from build123d import *

# Parameters (mm, degrees)
SKETCH1_W           = 126
SKETCH1_H           = 90
BOSS_EXTRUDE1_DEPTH = 3
BOSS_EXTRUDE2_DEPTH = 177
SKETCH3_W           = 126
SKETCH3_H           = 90
BOSS_EXTRUDE3_DEPTH = 3
FILLET1_R           = 10
SKETCH5_R           = 3
CUT_EXTRUDE1_DEPTH  = 5
SKETCH6_W           = 22.5
SKETCH6_H           = 13.5
SKETCH6_W_2         = 15
SKETCH6_H_2         = 10
CUT_EXTRUDE2_DEPTH  = 3
SKETCH7_W           = 180
SKETCH7_H           = 180
BOSS_EXTRUDE5_DEPTH = 3
SKETCH8_OUTSIDE_W   = 236
SKETCH8_OUTSIDE_H   = 146
CUT_EXTRUDE3_DEPTH  = 181
SKETCH9_W           = 120
SKETCH9_H           = 87
CUT_EXTRUDE4_DEPTH  = 181
SKETCH11_W          = 10
SKETCH11_H          = 3
BOSS_EXTRUDE6_DEPTH = 10
SKETCH12_R          = 1.7
CUT_EXTRUDE5_DEPTH  = 10
SKETCH13_R          = 1.7
CUT_EXTRUDE6_DEPTH  = 10
SKETCH16_W          = 60
SKETCH16_H          = 45
SKETCH16_W_2        = 55.136481679
SKETCH16_H_2        = 30
SKETCH16_W_3        = 50
SKETCH16_W_4        = 57.73113964
SKETCH16_W_5        = 14.594951033
SKETCH16_W_6        = 24.912721932
SKETCH16_H_3        = 36.48422414
BOSS_EXTRUDE7_DEPTH = 5
SKETCH15_R          = 4.75
SKETCH15_R_2        = 3
SKETCH15_R_3        = 3.6
SKETCH15_R_4        = 4.6
SKETCH15_R_5        = 4.7
SKETCH15_W          = 22.5
SKETCH15_H          = 13.5
CUT_EXTRUDE7_DEPTH  = 7.5
FILLET3_R           = 2.27
SKETCH17_W          = 54
SKETCH17_H          = 180
CUT_EXTRUDE8_DEPTH  = 10
BOSS_EXTRUDE8_DEPTH = 2
SKETCH19_R          = 1.7
CUT_EXTRUDE9_DEPTH  = 12
SKETCH20_R          = 1.7
CUT_EXTRUDE10_DEPTH = 12


with BuildPart() as part:
    # Sketch1 → Boss-Extrude1 (new body)
    with BuildSketch(Plane.XY):
        with Locations((63, -45)):
            Rectangle(SKETCH1_W, SKETCH1_H)
    extrude(amount=BOSS_EXTRUDE1_DEPTH)

    # Sketch2 → Boss-Extrude2 (add)
    with BuildSketch(Plane(origin=(0, 0, 0), x_dir=(-1, 0, 0), z_dir=(0, 0, -1))):
        Polygon((-126, -90), (-126, 0), (0, 0), (0, -90), (-3, -90), (-3, -3), (-123, -3), (-123, -90), align=None)
    extrude(amount=-BOSS_EXTRUDE2_DEPTH)

    # Sketch3 → Boss-Extrude3 (add)
    with BuildSketch(Plane.XY.offset(177)):
        with Locations((63, -45)):
            Rectangle(SKETCH3_W, SKETCH3_H)
    extrude(amount=BOSS_EXTRUDE3_DEPTH)

    # Fillet1
    fillet1_edges = [part.edges().sort_by_distance(p)[0] for p in [
        (63, -3, 3),
        (63, -3, 177),
        (63, 0, 0),
        (63, 0, 180),
    ]]
    fillet(fillet1_edges, radius=FILLET1_R)

    # Sketch5 → Cut-Extrude1 (cut)
    with BuildSketch(Plane.ZY.offset(2)):
        with Locations((154.879918412, -80.109384213)):
            Circle(SKETCH5_R)
        with Locations((163.20022023, -80.109384213)):
            Circle(SKETCH5_R)
    extrude(amount=-CUT_EXTRUDE1_DEPTH, mode=Mode.SUBTRACT)

    # Sketch6 → Cut-Extrude2 (cut)
    with BuildSketch(Plane(origin=(126, 0, 0), x_dir=(0, 0, -1), z_dir=(1, 0, 0))):
        with Locations((-31.25, -25.595398102)):
            Rectangle(SKETCH6_W, SKETCH6_H)
        with Locations((-30.5, -72.125177246)):
            Rectangle(SKETCH6_W_2, SKETCH6_H_2)
    extrude(amount=-CUT_EXTRUDE2_DEPTH, mode=Mode.SUBTRACT)

    # Sketch7 → Boss-Extrude5 (add)
    with BuildSketch(Plane(origin=(0, -90, 0), x_dir=(-1, 0, 0), z_dir=(0, -1, 0))):
        with Locations((-90, -90)):
            Rectangle(SKETCH7_W, SKETCH7_H)
    extrude(amount=-BOSS_EXTRUDE5_DEPTH)

    # Sketch8 outside → Cut-Extrude3 (cut, through all)
    with BuildSketch(Plane.ZY):
        with Locations((90, -45)):
            Rectangle(SKETCH8_OUTSIDE_W, SKETCH8_OUTSIDE_H)
        with BuildLine():
            Line((0, -79.898662722), (0, -90))
            Line((0, -90), (10.101337278, -90))
            Line((10.101337278, -90), (169.898662722, -90))
            Line((169.898662722, -90), (180, -90))
            Line((180, -90), (180, -79.898662722))
            Line((180, -79.898662722), (180, -10.101337278))
            ThreePointArc((180, -10.101337278), (177.04138681, -2.95861319), (169.898662722, 0))
            Line((169.898662722, 0), (10.101337278, 0))
            ThreePointArc((10.101337278, 0), (2.95861319, -2.95861319), (0, -10.101337278))
            Line((0, -10.101337278), (0, -79.898662722))
        make_face(mode=Mode.SUBTRACT)
    extrude(amount=-CUT_EXTRUDE3_DEPTH, mode=Mode.SUBTRACT)

    # Sketch9 → Cut-Extrude4 (cut, through all)
    with BuildSketch(Plane(origin=(0, 0, 0), x_dir=(-1, 0, 0), z_dir=(0, 0, -1))):
        with Locations((-63, -43.5)):
            Rectangle(SKETCH9_W, SKETCH9_H)
    extrude(amount=-CUT_EXTRUDE4_DEPTH, mode=Mode.SUBTRACT)

    # Sketch11 → Boss-Extrude6 (add)
    with BuildSketch(Plane(origin=(0, -87, 0), x_dir=(1, 0, 0), z_dir=(0, 1, 0))):
        with Locations((38, -178.5)):
            Rectangle(SKETCH11_W, SKETCH11_H)
        with Locations((88, -178.5)):
            Rectangle(SKETCH11_W, SKETCH11_H)
        with Locations((38, -1.5)):
            Rectangle(SKETCH11_W, SKETCH11_H)
        with Locations((88, -1.5)):
            Rectangle(SKETCH11_W, SKETCH11_H)
    extrude(amount=BOSS_EXTRUDE6_DEPTH)

    # Sketch12 → Cut-Extrude5 (cut)
    with BuildSketch(Plane(origin=(0, 0, 0), x_dir=(-1, 0, 0), z_dir=(0, 0, -1))):
        with Locations((-88, -82)):
            Circle(SKETCH12_R)
        with Locations((-38, -82)):
            Circle(SKETCH12_R)
    extrude(amount=-CUT_EXTRUDE5_DEPTH, mode=Mode.SUBTRACT)

    # Sketch13 → Cut-Extrude6 (cut)
    with BuildSketch(Plane.XY.offset(180)):
        with Locations((38, -82)):
            Circle(SKETCH13_R)
        with Locations((88, -82)):
            Circle(SKETCH13_R)
    extrude(amount=-CUT_EXTRUDE6_DEPTH, mode=Mode.SUBTRACT)

    # Sketch16 → Boss-Extrude7 (add)
    with BuildSketch(Plane.ZY.offset(2)):
        with Locations((33.397799687, -29.5)):
            Rectangle(SKETCH16_W, SKETCH16_H)
        with Locations((33.81824084, -70)):
            Rectangle(SKETCH16_W_2, SKETCH16_H_2)
        with Locations((93.535533906, -30.5)):
            Rectangle(SKETCH16_W_3, SKETCH16_H)
        with Locations((92.012227586, -70)):
            Rectangle(SKETCH16_W_4, SKETCH16_H_2)
        with Locations((130.607764761, -69.962221636)):
            Rectangle(SKETCH16_W_5, SKETCH16_H_2)
        with Locations((165.153259598, -44.347490411)):
            Rectangle(SKETCH16_W_6, SKETCH16_H_3)
    extrude(amount=-BOSS_EXTRUDE7_DEPTH)

    # Sketch15 → Cut-Extrude7 (cut, symmetric)
    with BuildSketch(Plane.ZY.offset(2)):
        with Locations((11.897799687, -25)):
            Circle(SKETCH15_R)
        with Locations((35.120412136, -25)):
            Circle(SKETCH15_R_2)
        with Locations((55.547244011, -25)):
            Circle(SKETCH15_R_3)
        with Locations((93.316630751, -36.188493445)):
            Circle(SKETCH15_R_4)
        with Locations((12.826376296, -70.752206375)):
            Circle(SKETCH15_R_3)
        with Locations((54.826376296, -70.752206375)):
            Circle(SKETCH15_R_3)
        with Locations((34.603168291, -70.752206375)):
            Circle(SKETCH15_R_4)
        with Locations((35.201614473, -42.050293137)):
            Circle(SKETCH15_R_4)
        with Locations((112.872652377, -74.126778902)):
            Circle(SKETCH15_R_3)
        with Locations((130.71133323, -74.126778902)):
            Circle(SKETCH15_R_3)
        with Locations((139.753590628, -46.167682179)):
            Circle(SKETCH15_R_5)
        with Locations((165.243179484, -54.550293137)):
            Circle(SKETCH15_R_3)
        with Locations((165.243179484, -38.990832132)):
            Circle(SKETCH15_R_2)
        with Locations((84.43777437, -74.416080578)):
            Rectangle(SKETCH15_W, SKETCH15_H)
    extrude(amount=CUT_EXTRUDE7_DEPTH, both=True, mode=Mode.SUBTRACT)

    # Fillet3
    fillet3_edges = [part.edges().sort_by_distance(p)[0] for p in [
        (-1, -52, 3.397799687),
        (-1, -7, 3.397799687),
        (-1, -7, 63.397799687),
        (-1, -52, 63.397799687),
        (-1, -85, 6.25),
        (-1, -55, 6.25),
        (-1, -55, 61.386481679),
        (-1, -85, 61.386481679),
        (-1, -53, 68.535533906),
        (-1, -8, 68.535533906),
        (-1, -8, 118.535533906),
        (-1, -53, 118.535533906),
        (-1, -85, 63.146657766),
        (-1, -55, 63.146657766),
        (-1, -55, 120.877797406),
        (-1, -85, 120.877797406),
        (-1, -84.962221636, 123.310289245),
        (-1, -54.962221636, 123.310289245),
        (-1, -54.962221636, 137.905240278),
        (-1, -84.962221636, 137.905240278),
        (-1, -62.589602481, 152.696898632),
        (-1, -26.105378341, 152.696898632),
        (-1, -26.105378341, 177.609620564),
        (-1, -62.589602481, 177.609620564),
    ]]
    fillet(fillet3_edges, radius=FILLET3_R)

    # Sketch17 → Cut-Extrude8 (cut)
    with BuildSketch(Plane(origin=(0, -87, 0), x_dir=(1, 0, 0), z_dir=(0, 1, 0))):
        with Locations((153, -90)):
            Rectangle(SKETCH17_W, SKETCH17_H)
    extrude(amount=-CUT_EXTRUDE8_DEPTH, mode=Mode.SUBTRACT)

    # Sketch18 → Boss-Extrude8 (add)
    with BuildSketch(Plane.ZY):
        with BuildLine():
            Line((129, -5), (171, -5))
            ThreePointArc((171, -5), (173.828427125, -6.171572875), (175, -9))
            Line((175, -9), (175, -19))
            ThreePointArc((175, -19), (173.828427125, -21.828427125), (171, -23))
            Line((171, -23), (129, -23))
            ThreePointArc((129, -23), (126.171572875, -21.828427125), (125, -19))
            Line((125, -19), (125, -9))
            ThreePointArc((125, -9), (126.171572875, -6.171572875), (129, -5))
        make_face()
    extrude(amount=BOSS_EXTRUDE8_DEPTH)

    # Sketch19 → Cut-Extrude9 (cut)
    with BuildSketch(Plane.ZY.offset(2)):
        with Locations((98.68777437, -74.666080578)):
            Circle(SKETCH19_R)
        with Locations((70.18777437, -74.666080578)):
            Circle(SKETCH19_R)
    extrude(amount=-CUT_EXTRUDE9_DEPTH, mode=Mode.SUBTRACT)

    # Sketch20 → Cut-Extrude10 (cut)
    with BuildSketch(Plane(origin=(126, 0, 0), x_dir=(0, 0, -1), z_dir=(1, 0, 0))):
        with Locations((-17, -25.845398102)):
            Circle(SKETCH20_R)
        with Locations((-45.5, -25.845398102)):
            Circle(SKETCH20_R)
    extrude(amount=-CUT_EXTRUDE10_DEPTH, mode=Mode.SUBTRACT)


solid = part.part
CAD build for the part. Positions are in the model's coordinates, mm. A direction names the side the tool comes from. Coordinates: 2 decimals unless noted, no trailing zeros. Loops run counter-clockwise (first coordinate to the right, second up) from the corner with the lowest first, then second, coordinate; pieces in that order, holes last. Notation, with made-up numbers: (88, 78.5) - (128, 78.5) arc R14 ccw to (128, 86.5) - close; hole circle Ø11 at (-13.75, -28). An arc over 180 degrees is marked (long way). Write item = value, one per line. Start each with the question number.
Q1. Which spindle directions (+Z, -Z, +X, -X, +Y, -Y) get a long thin tool onto all of the face, cutting with end or side? Do faces 1 (the cylindrical face through (-0.986, -6.203, 126.141)), 2 (the flat face through (0, -81.166, 84)), 3 (the flat face through (3, -44, 89)). Say none if no direction does.
Q2. Cut at A-A, the plane z = 132. List the corners of the cut face in (x, y).
Q3. Cut at B-B, the plane x = 107.5. List the corners of the cut face in (y, z).
Q4. Drill centre lines: L1, parallel to X at y = -82, z = 2; L2, parallel to X at y = -59, z = 139; L3, parallel to X at y = -67, z = 60. Where is each one in solid material? Low to high.
Q5. Flat gauge pins, fed straight in: pin 1 Ø8 at (x, z) = (37, 40) entering from +Y; pin 2 Ø1.5 at (x, z) = (88, 2) entering from +Y; pin 3 Ø0.6 at (x, z) = (-0.5, 30.5) entering from +Y; pin 4 Ø8.5 at (y, z) = (-74.13, 130.71) entering from -X. Where does each tip first touch, or does it go through?
Q6. Pull direction Z, two halves, no side cores. Call faces 4 (the flat face through (64, -87, 89)), 5 (the flat face through (64, -90, 89)), 6 (the cylindrical face through (0.46, -24.84, 51.95)), 7 (the cylindrical face through (1.48, -2.88, 3.04)): pulls with the +Z half, pulls with the -Z half, needs draft (parallel to the pull), parting line crosses it, or undercut.
Computed:
q1.face_1 = -X, +Y
q1.face_2 = -X
q1.face_3 = +Z, -Z, +Y
q2.outline = (-2, -84.96) - (0, -84.96) - (0, -90) - (126, -90) - (126, 0) - (123, 0) - (123, -87) - (3, -87) - (3, -77.49) - (-2, -77.49) - close; (-2, -70.77) - (3, -70.77) - (3, 0) - (0, 0) - (0, -5) - (-2, -5) - (-2, -23) - (0, -23) - (0, -54.96) - (-2, -54.96) - close
q3.outline = (-90, 0) - (-87, 0) - (-87, 180) - (-90, 180) - close
q4.L1 = 0 to 3, 33 to 36.3, 39.7 to 43, 83 to 86.3, 89.7 to 93, 123 to 126
q4.L2 = 0 to 3, 123 to 126
q4.L3 = -2 to 3, 123 to 126
q5.pin_1 = -87
q5.pin_2 = -77
q5.pin_3 = -7
q5.pin_4 = -2
q6.face_4 = undercut
q6.face_5 = needs draft
q6.face_6 = undercut
q6.face_7 = pulls with the -Z half
